Read the model definition and answer for the solid it produces. Units are mm, in the model's axes. Coordinates: 2 decimals unless noted, no trailing zeros. Write each loop counter-clockwise with the first axis right and the second up, starting at its lowest first coordinate (ties: lowest second). Pieces come first, ordered by that corner, then holes. Notation, with made-up numbers: (49.25, 47) - (63.25, 47) arc R17 ccw to (63.25, 62) - close; hole circle Ø3 at (68.25, 51). An arc over 180 degrees is marked (long way). Use a Markdown table: item, result.
Autodesk Inventor part; units mm, degrees
ref_plane "YZ Plane" through (0, 0, 0) normal (1, 0, 0) x (0, 1, 0)
ref_plane "XZ Plane" through (0, 0, 0) normal (0, 1, 0) x (-1, 0, 0)
ref_plane "XY Plane" through (0, 0, 0) normal (0, 0, 1) x (1, 0, 0)
sketch "Sketch1" plane through (0, 0, 0) normal (0, 0, 1) x (1, 0, 0)
  circle A0 centre (0, 0) radius 2.0955 construction
  circle A1 centre (31.2825, 19.6012) radius 7.2 construction
  circle A2 centre (43.3748, -2.7357) radius 2.15 construction
  circle A3 centre (31.2825, 19.6012) radius 31.75 construction
  circle A4 centre (43.3748, -2.7357) radius 2.032 construction
  line L0 (31.2825, 19.6012) -> (31.2825, -12.1488) construction
  circle A5 centre (31.2825, -12.1488) radius 2.032 construction
  line L1 (31.2825, 19.6012) -> (62.5502, 25.1146) construction
  line L2 (31.2825, 19.6012) -> (63.0325, 19.6012) construction
  circle A6 centre (62.5502, 25.1146) radius 2.032
  arc A7 (67.7804, 21.5135) -> (64.041, 31.2871) centre (62.5502, 25.1146) ccw
  circle A8 centre (0, 0) radius 2.032
  arc A9 (-5.017, 3.8926) -> (3.4439, -5.335) centre (0, 0) ccw
  arc A10 (45.62, -8.6755) -> (48.605, -6.3367) centre (43.3748, -2.7357) ccw
  circle A11 centre (22.0786, -10.7854) radius 2.032
  line L3 (48.605, -6.3367) -> (67.7804, 21.5135)
  arc A12 (35.755, 38.1188) -> (16.2316, 31.279) centre (31.2825, 19.6012) ccw
  line L4 (64.041, 31.2871) -> (35.755, 38.1188)
  line L5 (-5.017, 3.8926) -> (16.2316, 31.279)
  arc A13 (16.7437, -14.2294) -> (24.3239, -16.7253) centre (22.0786, -10.7854) ccw
  arc A14 (12.2228, -7.226) -> (3.4439, -5.335) centre (6.8878, -10.67) ccw
  line L6 (16.7437, -14.2294) -> (12.2228, -7.226)
  line L7 (45.9985, -8.5324) -> (24.3239, -16.7253)
  line L8 (27.7013, 17.6318) -> (32.3477, 15.7072)
  line L9 (27.7013, 17.6318) -> (27.7013, 17.6318)
  line L10 (32.3477, 15.7072) -> (27.7013, 17.6318)
  line L11 (32.3477, 15.7072) -> (32.3477, 15.7072)
  line L12 (33.1773, 16.0509) -> (35.1019, 20.6973)
  line L13 (33.1773, 16.0509) -> (33.1773, 16.0509)
  line L14 (35.1019, 20.6973) -> (33.1773, 16.0509)
  line L15 (35.1019, 20.6973) -> (35.1019, 20.6973)
  line L16 (34.7583, 21.5269) -> (30.1119, 23.4515)
  line L17 (34.7583, 21.5269) -> (34.7583, 21.5269)
  line L18 (30.1119, 23.4515) -> (34.7583, 21.5269)
  line L19 (30.1119, 23.4515) -> (30.1119, 23.4515)
  line L20 (29.2822, 23.1079) -> (27.3576, 18.4615)
  line L21 (29.2822, 23.1079) -> (29.2822, 23.1079)
  line L22 (27.3576, 18.4615) -> (29.2822, 23.1079)
  line L23 (27.3576, 18.4615) -> (27.3576, 18.4615)
  line L24 (35.1019, 20.6973) -> (35.3449, 21.2839)
  line L25 (34.7583, 21.5269) -> (35.3449, 21.2839)
  line L26 (33.1773, 16.0509) -> (32.9343, 15.4642)
  line L27 (32.3477, 15.7072) -> (32.9343, 15.4642)
  line L28 (29.2822, 23.1079) -> (29.5252, 23.6945)
  line L29 (30.1119, 23.4515) -> (29.5252, 23.6945)
  line L30 (27.3576, 18.4615) -> (27.1146, 17.8748)
  line L31 (27.7013, 17.6318) -> (27.1146, 17.8748)
  point P0 (0, 0)
extrude "Plate1" add sketch "Sketch1" along normal blind 1.5875
sketch "Sketch2" plane through (0, 0, 1.5875) normal (0, 0, 1) x (1, 0, 0)
  arc A0 (-5.017, 3.8926) -> (3.4439, -5.335) centre (0, 0) ccw
  line L0 (-5.017, 3.8926) -> (16.2316, 31.279)
  arc A1 (35.755, 38.1188) -> (16.2316, 31.279) centre (31.2825, 19.6012) ccw
  line L1 (35.755, 38.1188) -> (64.041, 31.2871)
  arc A2 (67.7804, 21.5135) -> (64.041, 31.2871) centre (62.5502, 25.1146) ccw
  line L2 (67.7804, 21.5135) -> (48.605, -6.3367)
  arc A3 (45.62, -8.6755) -> (48.605, -6.3367) centre (43.3748, -2.7357) ccw
  line L3 (45.62, -8.6755) -> (24.3239, -16.7253)
  arc A4 (16.7437, -14.2294) -> (24.3239, -16.7253) centre (22.0786, -10.7854) ccw
  line L4 (16.7437, -14.2294) -> (12.2228, -7.226)
  arc A5 (12.2228, -7.226) -> (3.4439, -5.335) centre (6.8878, -10.67) ccw
  circle A6 centre (0, 0) radius 2.032
  circle A7 centre (22.0786, -10.7854) radius 2.032
  circle A8 centre (62.5502, 25.1146) radius 2.032
  line L5 (29.5252, 23.6945) -> (35.3449, 21.2839)
  line L6 (27.1146, 17.8748) -> (29.5252, 23.6945)
  line L7 (35.3449, 21.2839) -> (32.9343, 15.4642)
  line L8 (32.9343, 15.4642) -> (27.1146, 17.8748)
  point P0 (0, 0)
equation "\"d20\" = Thickness"
equation "\"BendRadius\" = Thickness"
equation "\"BendReliefWidth\" = Thickness"
equation "\"BendReliefDepth\" = 0.5 * Thickness"
equation "\"CornerReliefSize\" = 4 * Thickness"
equation "\"MinimumRemnant\" = 2 * Thickness"
equation "\"TransitionRadius\" = BendRadius"
equation "\"JacobiRadiusSize\" = BendRadius"
equation "\"GapSize\" = Thickness"
properties part number "Rear Vertical Odom Pod" material "Acetal Resin, White"
(1) A cutting plane is placed at B-B, the plane y = 0. Write down the section's boundary in (x, z), and give its area (3 significant figures).
Report:
| item | result |
|---|---|
| outline | (-6.35, 0) - (-2.03, 0) - (-2.03, 1.59) - (-6.35, 1.59) - close; (2.03, 0) - (52.97, 0) - (52.97, 1.59) - (2.03, 1.59) - close |
| area | 87.7 mm² |
(2) The mould has two halves that part along X. Classify faces 1 (the cylindrical face through (60.938, 26.351, 0.783)), 2 (the cylindrical face through (47.31, -7.72, 0.78)), 3 (the flat face through (31, 11, 0)): pulls with the +X half, pulls with the -X half, needs draft (parallel to the pull), parting line crosses it, or undercut.
Report:
| item | result |
|---|---|
| face 1 | undercut |
| face 2 | pulls with the +X half |
| face 3 | needs draft |
(3) Straight lines are drawn through the part: L1, parallel to Y at x = 0, z = 0.45; L2, parallel to Y at x = 63, z = 0.2; L3, parallel to X at y = 23, z = 1.25. For each, find the intervals that lie inside material, in ascending order.
Report:
| item | result |
|---|---|
| L1 | y = -6.35 to -2.03, 2.03 to 10.36 |
| L2 | y = 14.57 to 23.13, 27.1 to 31.54 |
| L3 | x = 9.81 to 29.24, 31.2 to 68.54 |
(4) A cutting plane is placed at A-A, the plane x = 0. Write down the section's boundary in (y, z).
Report:
| item | result |
|---|---|
| outline | (-6.35, 0) - (-2.03, 0) - (-2.03, 1.59) - (-6.35, 1.59) - close; (2.03, 0) - (10.36, 0) - (10.36, 1.59) - (2.03, 1.59) - close |
(5) A cutting plane is placed at D-D, the plane x = 53.5. Write down the section's boundary in (y, z).
Report:
| item | result |
|---|---|
| outline | (0.77, 0) - (33.83, 0) - (33.83, 1.59) - (0.77, 1.59) - close |
(6) A cutting plane is placed at C-C, the plane z = 0.45. Write down the section's boundary in (x, y) (1 decimal), and give its area (3 significant figures).
Report:
| item | result |
|---|---|
| outline | (-5, 3.9) arc R6.4 ccw to (3.4, -5.3) arc R6.3 cw to (12.2, -7.2) - (16.7, -14.2) arc R6.4 ccw to (24.3, -16.7) - (45.6, -8.7) arc R6.4 ccw to (48.6, -6.3) - (67.8, 21.5) arc R6.3 ccw to (64, 31.3) - (35.8, 38.1) arc R19 ccw to (16.2, 31.3) - close; hole circle Ø4.1 at (0, 0); hole circle Ø4.1 at (22.1, -10.8); hole (27.1, 17.9) - (27.7, 17.6) - (32.3, 15.7) - (32.9, 15.5) - (33.2, 16.1) - (35.1, 20.7) - (35.3, 21.3) - (34.8, 21.5) - (30.1, 23.5) - (29.5, 23.7) - (29.3, 23.1) - (27.4, 18.5) - close; hole circle Ø4.1 at (62.6, 25.1) |
| area | 2,540 mm² |
